Autodesk Inventor part; units mm, degrees
ref_plane "РабПлоскость2" through (-464.2239, 154.5996, -124.0538) normal (0, 1, 0) x (0, 0, 1)
ref_plane "YZ Plane" through (0, 0, 0) normal (1, 0, 0) x (0, 1, 0)
ref_plane "XZ Plane" through (0, 0, 0) normal (0, 1, 0) x (-1, 0, 0)
ref_plane "РабПлоскость1" through (-329.2239, 210.3045, -11.0538) normal (0, -1, 0) x (1, 0, 0)
sketch "Эскиз1" plane through (-329.2239, 210.3045, -11.0538) normal (0, -1, 0) x (1, 0, 0)
  line L0 (-46.5606, -73) -> (-52.5606, -73)
  line L1 (-52.5606, -73) -> (-52.5606, -43)
  line L2 (-52.5606, -43) -> (-46.5606, -43)
  line L3 (-46.5606, -43) -> (-46.5606, -73)
  line L4 (-23.55, -78) -> (-51.55, -78)
  point P0 (329.2239, 11.0538)
  dimension "d0" = 6
  dimension "d1" = 30
  dimension "d2" = 5
ref_plane "РабПлоскость2" through (-464.2239, 154.5996, -124.0538) normal (0, 1, 0) x (0, 0, 1)
extrude "Выдавливание1" add sketch "Эскиз1" along normal blind 55.705 and the other way blind 5.645
sketch "Эскиз2" plane through (-375.7846, 215.9495, -54.0538) normal (1, 0, 0) x (0, 0, -1)
  line L0 (30, 0) -> (30, -61.35)
  line L1 (30, -30.675) -> (0, -30.675)
  line L2 (0, 0) -> (0, -61.35)
  line L3 (30, 0) -> (23, 0)
  line L4 (23, 0) -> (23, 5)
  line L5 (23, 5) -> (30, 5)
  line L6 (30, 5) -> (30, 0)
  line L7 (0, 0) -> (7, 0)
  line L8 (7, 0) -> (7, 5)
  line L9 (7, 5) -> (0, 5)
  line L10 (0, 5) -> (0, 0)
  line L11 (18.25, -4.5) -> (11.75, -4.5)
  line L12 (11.75, -4.5) -> (11.75, -7)
  line L13 (11.75, -7) -> (18.25, -7)
  line L14 (18.25, -7) -> (18.25, -4.5)
  line L15 (13.25, -9.1998) -> (16.75, -9.1998)
  line L16 (16.75, -9.1998) -> (16.75, 2.1998)
  line L17 (16.75, 2.1998) -> (13.25, 2.1998)
  line L18 (13.25, 2.1998) -> (13.25, -9.1998)
  line L19 (13.25, -9.1998) -> (16.75, 2.1998) construction
  line L20 (16.75, -9.1998) -> (13.25, 2.1998) construction
  line L21 (30, -61.35) -> (23, -61.35)
  line L22 (23, -61.35) -> (23, -66.35)
  line L23 (23, -66.35) -> (30, -66.35)
  line L24 (30, -66.35) -> (30, -61.35)
  line L25 (0, -61.35) -> (7, -61.35)
  line L26 (7, -61.35) -> (7, -66.35)
  line L27 (7, -66.35) -> (0, -66.35)
  line L28 (0, -66.35) -> (0, -61.35)
  line L29 (18.25, -54.35) -> (18.25, -56.85)
  line L30 (16.75, -63.5498) -> (13.25, -63.5498)
  line L31 (16.75, -52.1502) -> (16.75, -63.5498)
  line L32 (13.25, -52.1502) -> (16.75, -52.1502)
  line L33 (13.25, -52.1502) -> (16.75, -63.5498) construction
  line L34 (13.25, -63.5498) -> (13.25, -52.1502)
  line L35 (16.75, -52.1502) -> (13.25, -63.5498) construction
  line L36 (18.25, -56.85) -> (11.75, -56.85)
  line L37 (11.75, -56.85) -> (11.75, -54.35)
  line L38 (11.75, -54.35) -> (18.25, -54.35)
  point P0 (-54.0538, -215.9495)
  point P1 (0, -55.705)
  point P2 (30, -55.705)
  point P3 (15, -3.5)
  point P4 (16.75, -7)
  point P5 (16.75, -4.5)
  point P6 (13.25, -4.5)
  point P7 (13.25, -7)
  point P8 (15, -57.85)
  point P9 (16.75, -56.85)
  point P10 (16.75, -54.35)
  point P11 (13.25, -54.35)
  point P12 (13.25, -56.85)
  dimension "d23" = 5
  dimension "d24" = 7
  dimension "d25" = 7
extrude "Выдавливание2" add sketch "Эскиз2" against normal blind 6 contours L3 L4 L5 L6 | L10 L9 L8 L7 | L24 L23 L22 L21 | L25 L26 L27 L28
extrude "Выдавливание3" cut sketch "Эскиз2" against normal blind 6 contours L14 L13 L16 L11 | L16 L13 L18 L11 | L11 L18 L17 L16 | L18 L13 L12 L11 | L16 L15 L18 L13 | L29 L36 L31 L38 | L38 L34 L32 L31 | L31 L36 L34 L38 | L31 L30 L34 L36 | L34 L36 L37 L38
sketch "Эскиз6" plane through (-381.7846, 149.5995, -84.0538) normal (-1, 0, 0) x (0, 0, 1)
  line L0 (19.8477, 42.2969) -> (9.8477, 42.2969)
  line L1 (9.8477, 46.2969) -> (19.8477, 46.2969)
  line L2 (19.8477, 46.2969) -> (19.8477, 42.2969)
  line L3 (9.8477, 42.2969) -> (9.8477, 46.2969)
  point P0 (84.0538, -149.5995)
extrude "Выдавливание5" cut sketch "Эскиз6" against normal blind 6
properties part number "стенка 2"
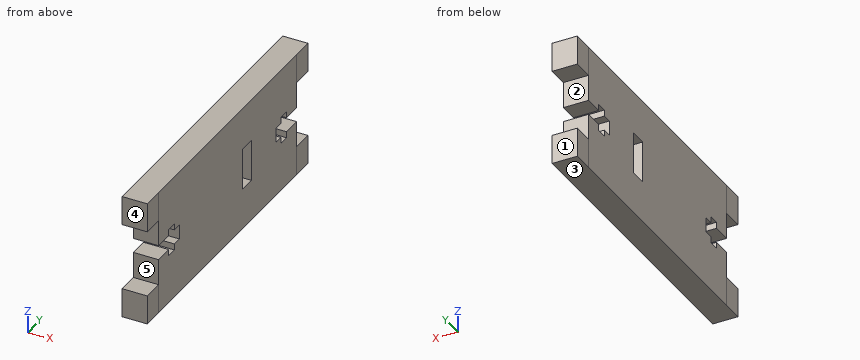
Geometry: final body of the model. Coordinates: model frame, mm. Face numbers are marked on the shaded views. A direction names the side the tool comes from. Coordinates: 2 decimals unless noted, no trailing zeros. Order: outer loops, then holes, each group sorted by start corner. A loop starts at its lowest first (then second) coordinate and runs counter-clockwise, first axis right, second up. Notation, with made-up numbers: (41.25, -4.5) - (51.25, -4.5) arc R23 ccw to (51.25, 19.5) - close; hole circle Ø2 at (48.25, 9.25). An arc over 180 degrees is marked (long way). Return JSON: item names as keys, results as strings. Group by question number.
1. Cut plane A-A (z = -70). Output: boundary loops of the cut face in (x, y), plus the area to 3 significant figures.
2. Set-up query: the marked faces 4 and 5. Return all of +Z, -Z, +X, -X, +Y, -Y with unobstructed straight access to the full face (end or side cutting, diameter ignored); none if empty.
3. Pin query (flat end, axial travel): pin 1 (0.8 mm diameter, centred on x = -380, z = -66.5, fed in from -Y); pin 2 (3 mm diameter, centred on x = -379, z = -70.5, fed in from +Y). Return the tip coordinate at first contact, or that it passes through.
4. Cut plane B-B (z = -63.25). Output: boundary loops of the cut face in (x, y), plus the area to 3 significant figures.
5. Pull-direction query (Z, two-part tool) for the marked faces 1, 2 and 3; classes: pulls with the +Z half, pulls with the -Z half, needs draft (parallel to the pull), parting line crosses it, or undercut.
6. Material intervals for line 1 along Y through (x, z) = (-378, -66.25); line 2 along Y through (x, z) = (-377, -65); line 3 along Z through (x, y) = (-380.5, 157.5), sorted ascending. Write a range as [from, to].
Resolved:
{
 "1": {"outline": "(-381.78, 163.8) - (-375.78, 163.8) - (-375.78, 191.9) - (-381.78, 191.9) - close; (-381.78, 195.9) - (-375.78, 195.9) - (-375.78, 206.75) - (-381.78, 206.75) - close", "area": "234 mm²"},
 "2": {"face 4": "+Z, -Z, +X, -X, -Y", "face 5": "+X, -X, -Y"},
 "3": {"pin 1": "stops at y = 154.6", "pin 2": "stops at y = 215.95"},
 "4": {"outline": "(-381.78, 154.6) - (-375.78, 154.6) - (-375.78, 215.95) - (-381.78, 215.95) - close", "area": "368 mm²"},
 "5": {"face 1": "needs draft", "face 2": "undercut", "face 3": "pulls with the -Z half"},
 "6": {"line 1": "y = [154.6, 159.1], [161.6, 191.9], [195.9, 208.95], [211.45, 215.95]", "line 2": "y = [154.6, 191.9], [195.9, 215.95]", "line 3": "z = [-84.05, -70.8], [-67.3, -54.05]"}
}
